The listing builds one solid part. Answer for the finished solid, in the listing's coordinates (mm). Face numbers are marked on the shaded views. A direction names the side the tool comes from. Give positions to 0.01 mm unless a question says otherwise; leave off trailing zeros. Write each loop counter-clockwise with the first axis right and the second up, starting at its lowest first coordinate (ties: lowest second). Pieces come first, ordered by that corner, then holes. Notation, with made-up numbers: (76, 30.25) - (118, 30.25) arc R12 ccw to (118, 36.25) - close; hole circle Ø5 at (41.25, 15.25). An arc over 180 degrees is marked (long way). One line per item, written item: value. Start each with the question number.
from build123d import *

# Parameters (mm, degrees)
SKETCH1_W               = 18
SKETCH1_H               = 18.3
BOSS_EXTRUDE1_DEPTH     = 3
SKETCH2_W               = 18
SKETCH2_H               = 4
BOSS_EXTRUDE3_DEPTH     = 8
SKETCH3_R               = 1.75
CUT_EXTRUDE2_DEPTH      = 20
CUT_EXTRUDE2_DEPTH_BACK = 13
FILLET1_R               = 1
FILLET2_R               = 1
FILLET3_R               = 1
SKETCH4_W               = 18
SKETCH4_H               = 18.3
BOSS_EXTRUDE4_DEPTH     = 1
SKETCH5_W               = 18
SKETCH5_H               = 40
BOSS_EXTRUDE5_DEPTH     = 5
SKETCH6_R               = 1.75
CUT_EXTRUDE4_DEPTH      = 5
FILLET4_R               = 1
FILLET5_R               = 1


with BuildPart() as part:
    # Sketch1 → Boss-Extrude1 (new body)
    with BuildSketch(Plane(origin=(0, 0, 0), x_dir=(1, 0, 0), z_dir=(0, 1, 0))):
        Rectangle(SKETCH1_W, SKETCH1_H)
    extrude(amount=BOSS_EXTRUDE1_DEPTH)

    # Sketch2 → Boss-Extrude3 (add)
    with BuildSketch(Plane(origin=(0, 3, 0), x_dir=(1, 0, 0), z_dir=(0, 1, 0))):
        with Locations((0, -7.15)):
            Rectangle(SKETCH2_W, SKETCH2_H)
        with Locations((0, 7.15)):
            Rectangle(SKETCH2_W, SKETCH2_H)
    extrude(amount=BOSS_EXTRUDE3_DEPTH)

    # Sketch3 → Cut-Extrude2 (cut, two sides)
    with BuildSketch(Plane(origin=(0, 0, 5.15), x_dir=(-1, 0, 0), z_dir=(0, 0, -1))) as cut_extrude2_sk:
        with Locations((-4.762, 7)):
            Circle(SKETCH3_R)
        with Locations((4.762, 7)):
            Circle(SKETCH3_R)
    extrude(amount=CUT_EXTRUDE2_DEPTH, mode=Mode.SUBTRACT)
    extrude(cut_extrude2_sk.sketch, amount=-CUT_EXTRUDE2_DEPTH_BACK, mode=Mode.SUBTRACT)

    # Fillet1
    fillet1_edges = [part.edges().sort_by_distance(p)[0] for p in [
        (0, 3, 5.15),
    ]]
    fillet(fillet1_edges, radius=FILLET1_R)

    # Fillet2
    fillet2_edges = [part.edges().sort_by_distance(p)[0] for p in [
        (0, 3, -5.15),
    ]]
    fillet(fillet2_edges, radius=FILLET2_R)

    # Fillet3
    fillet3_edges = [part.edges().sort_by_distance(p)[0] for p in [
        (0, 11, 5.15),
        (0, 11, -5.15),
    ]]
    fillet(fillet3_edges, radius=FILLET3_R)

    # Sketch4 → Boss-Extrude4 (add)
    with BuildSketch(Plane.XZ):
        Rectangle(SKETCH4_W, SKETCH4_H)
    extrude(amount=BOSS_EXTRUDE4_DEPTH)

    # Sketch5 → Boss-Extrude5 (add)
    with BuildSketch(Plane(origin=(0, -1, 0), x_dir=(-1, 0, 0), z_dir=(0, -1, 0))):
        Rectangle(SKETCH5_W, SKETCH5_H)
    extrude(amount=BOSS_EXTRUDE5_DEPTH)

    # Sketch6 → Cut-Extrude4 (cut)
    with BuildSketch(Plane.XZ.offset(6)):
        with Locations((4.5, 14.5)):
            Circle(SKETCH6_R)
        with Locations((-4.5, 14.5)):
            Circle(SKETCH6_R)
        with Locations((-4.5, -14.5)):
            Circle(SKETCH6_R)
        with Locations((4.5, -14.5)):
            Circle(SKETCH6_R)
    extrude(amount=-CUT_EXTRUDE4_DEPTH, mode=Mode.SUBTRACT)

    # Fillet4
    fillet4_edges = [part.edges().sort_by_distance(p)[0] for p in [
        (0, -1, -20),
    ]]
    fillet(fillet4_edges, radius=FILLET4_R)

    # Fillet5
    fillet5_edges = [part.edges().sort_by_distance(p)[0] for p in [
        (0, -1, 20),
    ]]
    fillet(fillet5_edges, radius=FILLET5_R)


solid = part.part
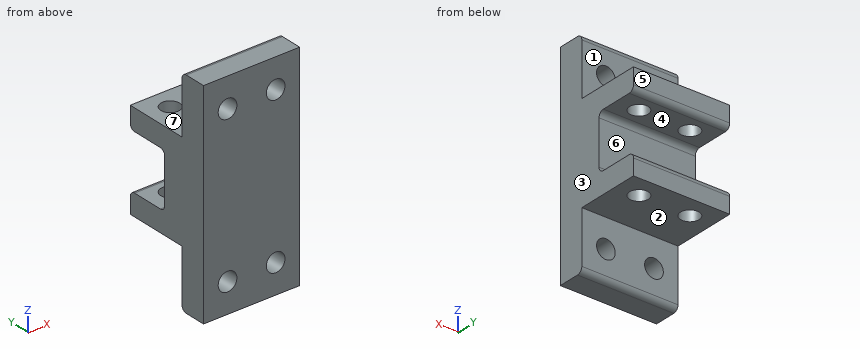
Item 1: Find section B-B on z = -14.5. Determine the outline of the cut face in (x, y).
Item 2: For the marked faces 1, 2 and 3, determine the directions among +Z, -Z, +X, -X, +Y, -Y from which every point of the face is accessible in a straight line to the end or side of a thin tool.
Item 3: Find section C-C on x = 5. Give the number of separate pieces and of enclosed holes in the cut face, plus the area to 3 significant figures.
Item 4: Find section D-D on x = -7.5. Determine the outline of the cut face in (y, z).
Item 5: The mould has two halves that part along Z. Classify the marked faces 4, 5, 6 and 7: +Z half, -Z half, draft (parallel to the pull), parting line (faces both ways), or undercut.
Item 6: Find section A-A on y = 7. Determine the outline of the cut face in (x, z), plus the area to 3 significant figures.
Item 7: Straight lines are drawn through the part: line 1 along X through (y, z) = (7, -8.3); line 2 along Z through (x, y) = (-4.5, -3.75); line 3 along Z through (x, y) = (-0.5, 7.25). For each, find the intervals that lie inside material, in ascending order.
Item 8: Each of these flat-tipped pins is pushed along its axis until it touches: pin 1 Ø6.5 at (x, z) = (-3.5, 1.5) entering from +Y; pin 2 Ø1 at (x, y) = (-1, 8) entering from +Z; pin 3 Ø1 at (x, z) = (-3, 16) entering from +Y. Where does it stop, or does it pass through?
Values:
1. outline: (-9, -6) - (-6.25, -6) - (-6.25, -1) - (-9, -1) - close; (-2.75, -6) - (2.75, -6) - (2.75, -1) - (-2.75, -1) - close; (6.25, -6) - (9, -6) - (9, -1) - (6.25, -1) - close
2. face 1: +Z, +X, -X, +Y
2. face 2: -Z, +X, -X, +Y
2. face 3: +Z, -Z, +X, +Y, -Y
3. separate pieces: 5
3. enclosed holes: 0
3. area: 275 mm^2
4. outline: (-6, -20) - (-2, -20) arc R1 ccw to (-1, -19) - (-1, -9.15) - (11, -9.15) - (11, -6.15) arc R1 ccw to (10, -5.15) - (4, -5.15) arc R1 cw to (3, -4.15) - (3, 4.15) arc R1 cw to (4, 5.15) - (10, 5.15) arc R1 ccw to (11, 6.15) - (11, 9.15) - (-1, 9.15) - (-1, 19) arc R1 ccw to (-2, 20) - (-6, 20) - close
5. face 4: undercut
5. face 5: draft
5. face 6: undercut
5. face 7: +Z half
6. outline: (-9, -9.15) - (-6.51, -9.15) - (-6.51, -5.15) - (-9, -5.15) - close; (-9, 5.15) - (-6.51, 5.15) - (-6.51, 9.15) - (-9, 9.15) - close; (-3.01, -9.15) - (3.01, -9.15) - (3.01, -5.15) - (-3.01, -5.15) - close; (-3.01, 5.15) - (3.01, 5.15) - (3.01, 9.15) - (-3.01, 9.15) - close; (6.51, -9.15) - (9, -9.15) - (9, -5.15) - (6.51, -5.15) - close; (6.51, 5.15) - (9, 5.15) - (9, 9.15) - (6.51, 9.15) - close
6. area: 88.0 mm^2
7. line 1: -9 to -6.51, -3.01 to 3.01, 6.51 to 9
7. line 2: -20 to -16.25, -12.75 to 12.75, 16.25 to 20
7. line 3: -9.15 to -5.15, 5.15 to 9.15
8. pin 1: y = 3.2
8. pin 2: z = 9.15
8. pin 3: y = -1
